The listing builds one solid part. Answer for the finished solid, in the listing's coordinates (mm). Coordinates: 2 decimals unless noted, no trailing zeros. Order: outer loops, then holes, each group sorted by start corner. A loop starts at its lowest first (then second) coordinate and runs counter-clockwise, first axis right, second up. Notation, with made-up numbers: (68.25, 34.5) -> (109.25, 34.5) arc R25 cw to (109.25, 73.5) -> close; hole circle Ø11 at (-34, 84). An arc over 180 degrees is marked (long way). Write item = value, one per line. Start each with the question number.
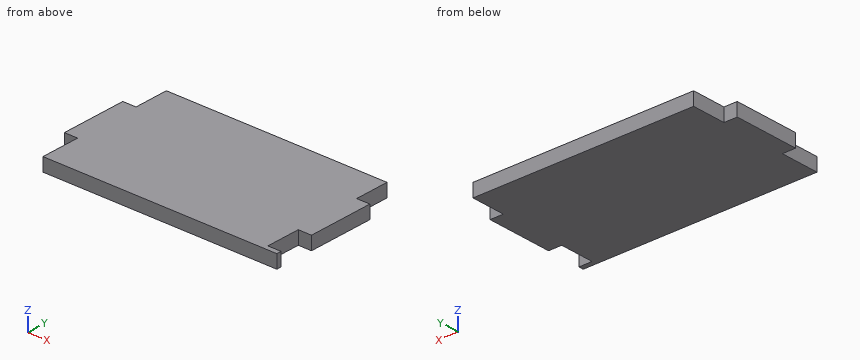
```python
from build123d import *

# Parameters (mm, degrees)
SKETCH1_W           = 56
SKETCH1_H           = 31.7
BOSS_EXTRUDE1_DEPTH = 3
SKETCH2_W           = 3
SKETCH2_H           = 7.8
CUT_EXTRUDE1_DEPTH  = 45.306907356
LPATTERN1_COUNT     = 2
LPATTERN1_PITCH     = 22.8
SKETCH3_W           = 3
SKETCH3_H           = 7.8
CUT_EXTRUDE2_DEPTH  = 45.306907356
LPATTERN2_COUNT     = 4
LPATTERN2_PITCH     = 22.8
SKETCH6_W           = 3
SKETCH6_H           = 1.1
CUT_EXTRUDE3_DEPTH  = 10


with BuildPart() as part:
    # Sketch1 → Boss-Extrude1 (new body)
    with BuildSketch(Plane.XY):
        with Locations((-12.993460648, 0.692013889)):
            Rectangle(SKETCH1_W, SKETCH1_H)
    extrude(amount=BOSS_EXTRUDE1_DEPTH)

    # Sketch2 → Cut-Extrude1 (cut, through all)
    with BuildSketch(Plane.XY.offset(3)):
        with Locations((-39.493460648, 12.642013889)):
            Rectangle(SKETCH2_W, SKETCH2_H)
    cut_extrude1 = extrude(amount=-CUT_EXTRUDE1_DEPTH, mode=Mode.SUBTRACT)

    # LPattern1: Cut-Extrude1 ×2
    with Locations(*[(0, -i * LPATTERN1_PITCH, 0) for i in range(1, LPATTERN1_COUNT)]):
        add(cut_extrude1, mode=Mode.SUBTRACT)

    # Sketch3 → Cut-Extrude2 (cut, through all)
    with BuildSketch(Plane.XY.offset(3)):
        with Locations((13.506539352, 12.642013889)):
            Rectangle(SKETCH3_W, SKETCH3_H)
    cut_extrude2 = extrude(amount=-CUT_EXTRUDE2_DEPTH, mode=Mode.SUBTRACT)

    # LPattern2: Cut-Extrude2 ×4
    with Locations(*[(0, -i * LPATTERN2_PITCH, 0) for i in range(1, LPATTERN2_COUNT)]):
        add(cut_extrude2, mode=Mode.SUBTRACT)

    # Sketch6 → Cut-Extrude3 (cut)
    with BuildSketch(Plane.XY.offset(3)):
        with Locations((-39.493460648, -14.607986111)):
            Rectangle(SKETCH6_W, SKETCH6_H)
    extrude(amount=-CUT_EXTRUDE3_DEPTH, mode=Mode.SUBTRACT)


solid = part.part
```
Item 1: Consider probe 1 along X at (y, z) = (11, 1.9). Determine where the line is inside the solid, lowest interval first.
Item 2: Section A-A, the plane z = 2.4 is taken. Give the vertices of the cut face in (x, y), then the cut area to 3 significant figures.
Item 3: Each of these flat-tipped pins is pushed along its axis until it touches: pin 1 (1.5 mm diameter, centred on y = -9.5, z = 1.5, fed in from +X); pin 2 (1.5 mm diameter, centred on y = -10, z = 1, fed in from -X); pin 3 (1.5 mm diameter, centred on x = 13, z = 2, fed in from +Y). Where does it stop, or does it pass through?
Item 4: Section B-B, the plane y = -7.5 is taken. Give the vertices of the cut face in (x, z), then the cut area to 3 significant figures.
A:
q1.probe_1 = -37.99 to 12.01
q2.outline = (-40.99, -6.26) -> (-37.99, -6.26) -> (-37.99, -15.16) -> (15.01, -15.16) -> (15.01, -14.06) -> (12.01, -14.06) -> (12.01, -6.26) -> (15.01, -6.26) -> (15.01, 8.74) -> (12.01, 8.74) -> (12.01, 16.54) -> (-37.99, 16.54) -> (-37.99, 8.74) -> (-40.99, 8.74) -> close
q2.area = 1,680 mm^2
q3.pin_1 = 12.01
q3.pin_2 = -37.99
q3.pin_3 = 8.74
q4.outline = (-37.99, 0) -> (12.01, 0) -> (12.01, 3) -> (-37.99, 3) -> close
q4.area = 150 mm^2
